```python
from build123d import *

# Parameters (mm, degrees)
MODEL_R             = 1.4605
MODEL_R_2           = 2
BOSS_EXTRUDE1_DEPTH = 1.27
SKETCH1_W           = 10
SKETCH1_H           = 24
CUT_EXTRUDE1_DEPTH  = 10


with BuildPart() as part:
    # Model → Boss-Extrude1 (new, symmetric)
    with BuildSketch(Plane.XY):
        with BuildLine():
            Line((-252.581304326, 70.3317), (-252.581304326, 25.8817))
            Line((-252.581304326, 25.8817), (-290.681304326, -12.2183))
            Line((-290.681304326, -12.2183), (-290.681304326, -50.3183))
            Line((-290.681304326, -50.3183), (-258.931304326, -82.0683))
            Line((-258.931304326, -82.0683), (-258.931304326, -139.2183))
            Line((-258.931304326, -139.2183), (-290.681304326, -170.9683))
            Line((-290.681304326, -170.9683), (-290.681304326, -190.0183))
            ThreePointArc((-290.681304326, -190.0183), (-288.821432386, -194.508428061), (-284.331304326, -196.3683))
            Line((-284.331304326, -196.3683), (-265.281304326, -196.3683))
            Line((-265.281304326, -196.3683), (-227.181304326, -158.2683))
            Line((-227.181304326, -158.2683), (-23.981304326, -158.2683))
            Line((-23.981304326, -158.2683), (14.118695674, -196.3683))
            Line((14.118695674, -196.3683), (33.168695674, -196.3683))
            ThreePointArc((33.168695674, -196.3683), (37.658823735, -194.508428061), (39.518695674, -190.0183))
            Line((39.518695674, -190.0183), (39.518695674, -170.9683))
            Line((39.518695674, -170.9683), (7.768695674, -139.2183))
            Line((7.768695674, -139.2183), (7.768695674, -82.0683))
            Line((7.768695674, -82.0683), (22.457936385, -67.37905929))
            Line((22.457936385, -67.37905929), (39.518695674, -50.3183))
            Line((39.518695674, -50.3183), (39.518695674, -12.2183))
            Line((39.518695674, -12.2183), (1.418695674, 25.8817))
            Line((1.418695674, 25.8817), (1.418695674, 70.3317))
            Line((1.418695674, 70.3317), (39.518695674, 108.4317))
            Line((39.518695674, 108.4317), (39.518695674, 127.4817))
            ThreePointArc((39.518695674, 127.4817), (37.658823735, 131.971828061), (33.168695674, 133.8317))
            Line((33.168695674, 133.8317), (14.118695674, 133.8317))
            Line((14.118695674, 133.8317), (-23.981304326, 95.7317))
            Line((-23.981304326, 95.7317), (-227.181304326, 95.7317))
            Line((-227.181304326, 95.7317), (-265.281304326, 133.8317))
            Line((-265.281304326, 133.8317), (-284.331304326, 133.8317))
            ThreePointArc((-284.331304326, 133.8317), (-288.821432386, 131.971828061), (-290.681304326, 127.4817))
            Line((-290.681304326, 127.4817), (-290.681304326, 108.4317))
            Line((-290.681304326, 108.4317), (-252.581304326, 70.3317))
        make_face()
        with Locations((-287.125304326, -190.6025)):
            Circle(MODEL_R, mode=Mode.SUBTRACT)
        with Locations((33.752895674, -190.6025)):
            Circle(MODEL_R, mode=Mode.SUBTRACT)
        with Locations((33.752895674, 130.2757)):
            Circle(MODEL_R, mode=Mode.SUBTRACT)
        with Locations((-287.125304326, 130.2757)):
            Circle(MODEL_R, mode=Mode.SUBTRACT)
        with Locations((-274.681304256, -57.7288)):
            Circle(MODEL_R, mode=Mode.SUBTRACT)
        with Locations((-254.681304256, -57.7288)):
            Circle(MODEL_R, mode=Mode.SUBTRACT)
        with Locations((23.518695604, -57.7288)):
            Circle(MODEL_R, mode=Mode.SUBTRACT)
        with Locations((3.518695604, -57.7288)):
            Circle(MODEL_R, mode=Mode.SUBTRACT)
        with Locations((23.518695604, -4.8078)):
            Circle(MODEL_R, mode=Mode.SUBTRACT)
        with Locations((3.518695604, -4.8078)):
            Circle(MODEL_R, mode=Mode.SUBTRACT)
        with Locations((-254.681304256, -4.8078)):
            Circle(MODEL_R, mode=Mode.SUBTRACT)
        with Locations((-274.681304256, -4.8078)):
            Circle(MODEL_R, mode=Mode.SUBTRACT)
        with Locations((-125.581304326, -12.2183)):
            Circle(MODEL_R_2, mode=Mode.SUBTRACT)
        with Locations((-125.581304326, -50.3183)):
            Circle(MODEL_R_2, mode=Mode.SUBTRACT)
        Polygon((-30.331304326, -145.5683), (-68.431304326, -107.4683), (-182.731304326, -107.4683), (-220.831304326, -145.5683), align=None, mode=Mode.SUBTRACT)
        Polygon((-220.831304326, 83.0317), (-182.731304326, 44.9317), (-68.431304326, 44.9317), (-30.331304326, 83.0317), align=None, mode=Mode.SUBTRACT)
        Polygon((-201.781304326, -69.3683), (-233.531304326, -37.6183), (-233.531304326, -24.9183), (-201.781304326, 6.8317), (-182.731304326, 6.8317), (-150.981304326, -24.9183), (-150.981304326, -37.6183), (-182.731304326, -69.3683), align=None, mode=Mode.SUBTRACT)
        Polygon((-100.181304326, -37.6183), (-100.181304326, -24.9183), (-68.431304326, 6.8317), (-49.381304326, 6.8317), (-17.631304326, -24.9183), (-17.631304326, -37.6183), (-49.381304326, -69.3683), (-68.431304326, -69.3683), align=None, mode=Mode.SUBTRACT)
    extrude(amount=BOSS_EXTRUDE1_DEPTH, both=True)

    # Sketch1 → Cut-Extrude1 (cut)
    with BuildSketch(Plane.XY.offset(1.27)):
        with Locations((-264.681304256, -57.7288)):
            Rectangle(SKETCH1_W, SKETCH1_H)
        with Locations((-264.681304256, -4.8078)):
            Rectangle(SKETCH1_W, SKETCH1_H)
        with Locations((13.518695604, -4.8078)):
            Rectangle(SKETCH1_W, SKETCH1_H)
        with Locations((13.518695604, -57.7288)):
            Rectangle(SKETCH1_W, SKETCH1_H)
    extrude(amount=-CUT_EXTRUDE1_DEPTH, mode=Mode.SUBTRACT)


solid = part.part
```
CAD build for the part. Positions are in the model's coordinates, mm. A direction names the side the tool comes from. Give positions to 0.01 mm unless a question says otherwise; leave off trailing zeros. Order: outer loops, then holes, each group sorted by start corner. A loop starts at its lowest first (then second) coordinate and runs counter-clockwise, first axis right, second up.
(1) Saw through at D-D, the plane z = 0.2. State how many separate pieces and enclosed holes the cut face has, then the cut area to 3 significant figures.
(2) Saw through at A-A, the plane x = -114.5. Give the cut face in (y, z).
(3) Tool access for faces 4 (the flat face through (-271.9, 89.65, 0.02)), 5 (the flat face through (-33.73, -8.82, 0.02)), 6 (the flat face through (-245.965, 114.515, 0.018)), 7 (the flat face through (20.202, 89.115, 0.018)): list every direction of +Z, -Z, +X, -X, +Y, -Y with a clear straight run to the whole face (end or side of a thin tool).
(4) Mould opens along Y. For faces 1 (the flat face through (-246.498, -177.585, 0.018)), 2 (the flat face through (-275, -66, 0)), 3 (the flat face through (-4.665, 115.048, 0.018)) say: released by +Y, released by -Y, zero draft, split by the parting line, or undercut.
(5) Drill centre lines: L1, parallel to Y at x = -136.5, z = 0.7; L2, parallel to X at y = 64, z = 0.95; L3, parallel to X at y = -63.5, z = 1.1. Where is each one in solid material? Low to high.
(6) Saw through at B-B, the plane y = 58. Give the cut face in (x, z), then the cut area to 3 significant figures.
(7) Flat gauge pins, fed straight in: pin 1 (1.3 mm diameter, centred on x = 12.5, z = 0.5, fed in from +Y); pin 2 (1 mm diameter, centred on y = 75, z = -0.5, fed in from +X); pin 3 (1.3 mm diameter, centred on y = -58.5, z = 0, fed in from +X). Where does each tip first touch, or does it go through?
(8) Saw through at C-C, the plane x = -209. Give the cut face in (y, z), then the cut area to 3 significant figures.
Results found:
1. separate pieces: 1
1. enclosed holes: 22
1. area: 57,400 mm2
2. outline: (-158.27, -1.27) - (-145.57, -1.27) - (-145.57, 1.27) - (-158.27, 1.27) - close; (-107.47, -1.27) - (44.93, -1.27) - (44.93, 1.27) - (-107.47, 1.27) - close; (83.03, -1.27) - (95.73, -1.27) - (95.73, 1.27) - (83.03, 1.27) - close
3. face 4: +Z, -Z, -X
3. face 5: +Z, -Z
3. face 6: +Z, -Z, +Y
3. face 7: +Z, -Z, +X
4. face 1: released by -Y
4. face 2: undercut
4. face 3: released by +Y
5. L1: y = -158.27 to -145.57, -107.47 to 44.93, 83.03 to 95.73
5. L2: x = -252.58 to -201.8, -49.36 to 1.42
5. L3: x = -277.5 to -269.68, -259.68 to -207.65, -176.86 to -74.3, -43.51 to 8.52, 18.52 to 26.34
6. outline: (-252.58, -1.27) - (-195.8, -1.27) - (-195.8, 1.27) - (-252.58, 1.27) - close; (-55.36, -1.27) - (1.42, -1.27) - (1.42, 1.27) - (-55.36, 1.27) - close
6. area: 288 mm2
7. pin 1: stops at y = 132.86
7. pin 2: stops at x = 6.59
7. pin 3: stops at x = 31.99
8. outline: (-158.27, -1.27) - (-145.57, -1.27) - (-145.57, 1.27) - (-158.27, 1.27) - close; (-133.74, -1.27) - (-62.15, -1.27) - (-62.15, 1.27) - (-133.74, 1.27) - close; (-0.39, -1.27) - (71.2, -1.27) - (71.2, 1.27) - (-0.39, 1.27) - close; (83.03, -1.27) - (95.73, -1.27) - (95.73, 1.27) - (83.03, 1.27) - close
8. area: 428 mm2
